Check sheet for the drawn part. Datum: minimum x, y, z corner. Units: mm. A direction names the side the tool comes from. Round coordinates to 2 decimals unless told otherwise and drop trailing zeros. Write each loop counter-clockwise with the first axis right and the second up, starting at its lowest first coordinate (ties: lowest second). Pieces come first, ordered by that corner, then holes. Notation, with made-up numbers: (4, 22.5) - (51, 22.5) arc R20 cw to (51, 55.5) - close; hole circle Ø10 at (23.25, 21). An arc over 180 degrees is marked (long way). Answer as a JSON object with one key per item and string values.
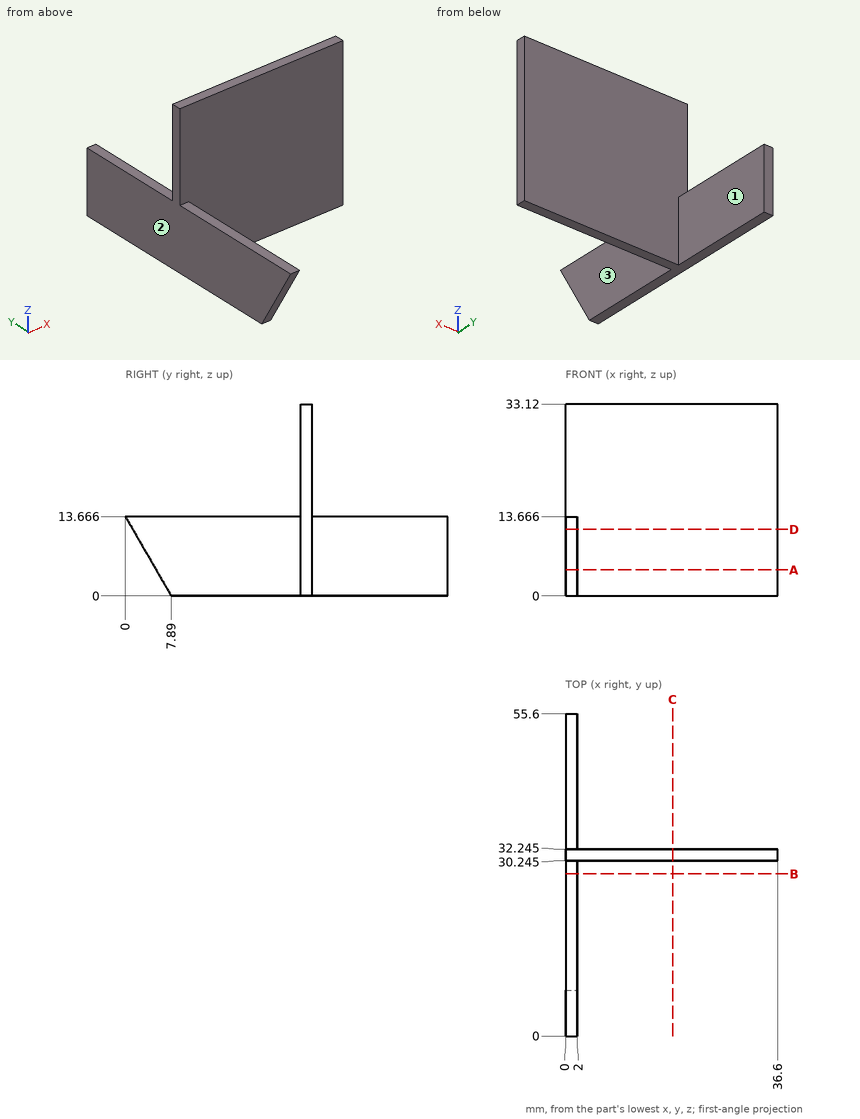
Q1. Section check C-C, the plane x = 18.5. Record the cut outline in (y, z) (3 decimals).
Geometry check:
{"outline": "(30.245, 0) - (32.245, 0) - (32.245, 33.12) - (30.245, 33.12) - close"}
Q2. Section check B-B, the plane y = 28. Record the cut outline in (x, z).
Geometry check:
{"outline": "(0, 0) - (2, 0) - (2, 13.67) - (0, 13.67) - close"}
Q3. Gauge pin test, flat ends, axial feed: P1, Ø16.5, axis at x = 17.5, z = 24, coming from the -Y side (3 decimals); P2, Ø7, axis at y = 44.5, z = 4.5, coming from the +X side; P3, Ø10, axis at x = 17, z = 13, coming from the +Y side (3 decimals); P4, Ø12, axis at y = 34, z = 20.5, coming from the -X side. Record the tip position at first contact, or that the pin passes through.
Geometry check:
{"P1": "stops at y = 30.245", "P2": "stops at x = 2", "P3": "stops at y = 32.245", "P4": "stops at x = 0"}
Q4. Section check D-D, the plane z = 11.5. Record the cut outline in (x, y) (1 decimal).
Geometry check:
{"outline": "(0, 1.3) - (2, 1.3) - (2, 30.2) - (36.6, 30.2) - (36.6, 32.2) - (2, 32.2) - (2, 55.6) - (0, 55.6) - close"}
Q5. Set-up check for the marked faces 1, 2 and 3: record each of +Z, -Z, +X, -X, +Y, -Y from which the full face is reachable in a straight line by a thin tool's end or side.
Geometry check:
{"face 1": "+Z, -Z, +X, +Y", "face 2": "+Z, -Z, -X, +Y, -Y", "face 3": "+Z, -Z, +X, -Y"}
Q6. Material ranges on line 1 along Y through (x, z) = (32.5, 25) (3 decimals); line 2 along X through (y, z) = (11.5, 5), recorded low to high. Write a range as [from, to].
Geometry check:
{"line 1": "y = [30.245, 32.245]", "line 2": "x = [0, 2]"}
Q7. Section check A-A, the plane z = 4.5. Record the cut outline in (x, y) (3 decimals), then the cut area to 3 significant figures.
Geometry check:
{"outline": "(0, 5.292) - (2, 5.292) - (2, 30.245) - (36.6, 30.245) - (36.6, 32.245) - (2, 32.245) - (2, 55.6) - (0, 55.6) - close", "area": "170 mm2"}
